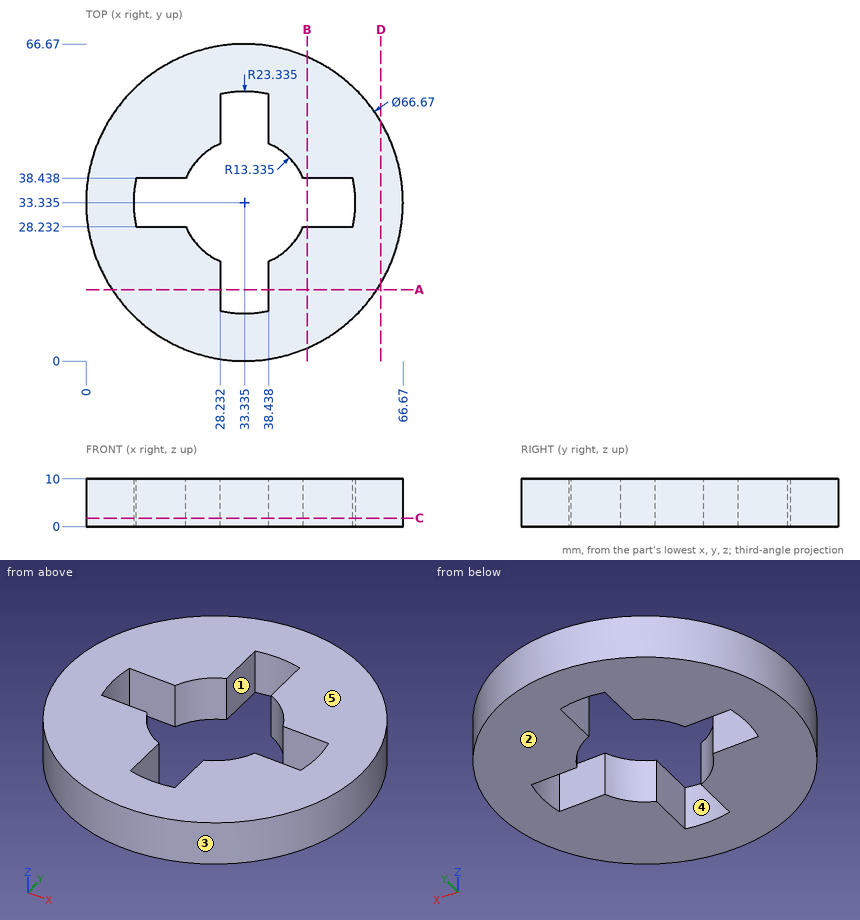
Part print with two shaded views. Sizes in mm from the minimum x, y, z corner. A direction names the side the tool comes from. Round coordinates to 2 decimals unless told otherwise and drop trailing zeros. Write each loop counter-clockwise with the first axis right and the second up, starting at its lowest first coordinate (ties: lowest second). Pieces come first, ordered by that corner, then holes. Notation, with made-up numbers: M 34.25,14 L 91.25,14 A32 ccw 91.25,52 Z; hole C 33.5,17.5 d8. An arc over 180 degrees is marked long. Put each result on its own line as item: value. Start each with the question number.
1) Saw through at C-C, the plane z = 1.75. Write the cut outline in (x, y) (3 decimals).
2) Drill centre lines: probe 1 along X at (y, z) = (22.5, 2.5); probe 2 along Y at (x, z) = (36, 7.5); probe 3 along X at (y, z) = (55.5, 4.75). Where is each one in solid material? Low to high. Write a range as [from, to].
3) Saw through at D-D, the plane x = 62. Write the cut outline in (y, z), and give its area (3 significant figures).
4) Saw through at A-A, the plane y = 15. Write the cut outline in (x, z).
5) Saw through at B-B, the plane x = 46.5. Write the cut outline in (y, z), and give its area (3 significant figures).
6) 3-axis set-ups, long thin cutter, end or side, ignore diameter. For the marked faces 1 and 2: which of +Z, -Z, +X, -X, +Y, -Y reach the whole face in a straight line?
7) Pull direction X, two halves, no side cores. Call the marked faces 3, 4 and 5: pulls with the +X half, pulls with the -X half, needs draft (parallel to the pull), parting line crosses it, or undercut.
8) Pin check, flat tips, straight feed: pin 1 Ø3 at (y, z) = (59.5, 7) entering from -X; pin 2 Ø3 at (y, z) = (50, 7.5) entering from -X; pin 3 Ø5 at (y, z) = (50, 2) entering from -X. Stop position of each tip, or through.
Resolved:
1. outline: C 33.335,33.335 d66.67; hole M 10.565,28.232 L 21.015,28.232 A13.335 ccw 28.232,21.015 L 28.232,10.565 A23.335 ccw 38.438,10.565 L 38.438,21.015 A13.335 ccw 45.655,28.232 L 56.105,28.232 A23.335 ccw 56.105,38.438 L 45.655,38.438 A13.335 ccw 38.438,45.655 L 38.438,56.105 A23.335 ccw 28.232,56.105 L 28.232,45.655 A13.335 ccw 21.015,38.438 L 10.565,38.438 A23.335 ccw Z
2. probe 1: [1.81, 25.56], [41.11, 64.86]
2. probe 2: [0.11, 10.15], [56.52, 66.56]
2. probe 3: [8.44, 28.23], [38.44, 58.23]
3. outline: M 16.32,0 L 50.35,0 L 50.35,10 L 16.32,10 Z
3. area: 340 mm²
4. outline: M 5.5,0 L 28.23,0 L 28.23,10 L 5.5,10 Z; M 38.44,0 L 61.17,0 L 61.17,10 L 38.44,10 Z
5. outline: M 2.71,0 L 28.23,0 L 28.23,10 L 2.71,10 Z; M 38.44,0 L 63.96,0 L 63.96,10 L 38.44,10 Z
5. area: 510 mm²
6. face 1: +Z, -Z
6. face 2: -Z, +X, -X, +Y, -Y
7. face 3: parting line crosses it
7. face 4: undercut
7. face 5: needs draft
8. pin 1: x = 10.91
8. pin 2: x = 3.65
8. pin 3: x = 3.16
